Source: CAD feature listing. Evaluate the final solid. Frame: model axes, mm. A direction names the side the tool comes from. Give positions to 0.01 mm unless a question says otherwise; leave off trailing zeros. Loops run counter-clockwise (first coordinate to the right, second up) from the corner with the lowest first, then second, coordinate; pieces in that order, holes last. Notation, with made-up numbers: (76.25, -2.5) - (114.25, -2.5) arc R11 ccw to (114.25, 11.5) - close; hole circle Ø11 at (26, -38). An arc over 180 degrees is marked (long way). Write each question's results on one line, items separated by ' | '. Start each with the question number.
(1) Pull-direction query (Y, two-part tool) for faces 1 (the flat face through (3, -1, 11.75)), 2 (the flat face through (-2.89, 8.54, 0.49)), 3 (the flat face through (8.84, -1.77, 0.49)); classes: pulls with the +Y half, pulls with the -Y half, needs draft (parallel to the pull), parting line crosses it, or undercut.
(2) Cut plane C-C on z = 22.5. Return the cut outline in (x, y), then the cut area to 3 significant figures.
(3) Cut plane B-B on z = 14. Return the cut outline in (x, y), then the cut area to 3 significant figures.
(4) Cut plane A-A on z = 9.75. Return the cut outline in (x, y), then the cut area to 3 significant figures.
(5) Material intervals for line 1 along Y through (x, z) = (0, 20.75); line 2 along Y through (x, z) = (0, 4.25); line 3 along Z through (x, y) = (3, 1.75), sorted ascending. Write a range as [from, to].
(6) Contact query for flat-ended pins moving along their axis: pin 1 (1.5 mm diameter, centred on y = -3.5, z = 6.5, fed in from +X); pin 2 (2 mm diameter, centred on x = -4.5, y = 7.5, fed in from +Z); pin 3 (9 mm diameter, centred on x = -1, y = -1.5, fed in from -Z); pin 4 (3.5 mm diameter, centred on x = 0, y = 0, fed in from +Z). Output: stop coordinate, or through.
(7) Reachability of faces 4 (the cylindrical face through (-1.08, 4.88, 21.44)), 5 (the cylindrical face through (0.75, 5.7, 6.3)), 6 (the flat face through (3.2, -8.97, 7.64)) from +Z, -Z, +X, -X, +Y, -Y: full face, straight path, thin tool, end or side. Return the list, or none.
Autodesk Inventor part; units mm, degrees
ref_plane "Work Plane1" through (0, 0, 16.51) normal (0, 0, 1) x (1, 0, 0)
ref_plane "YZ Plane" through (0, 0, 0) normal (1, 0, 0) x (0, 1, 0)
ref_plane "XZ Plane" through (0, 0, 0) normal (0, 1, 0) x (-1, 0, 0)
sketch "Sketch1" plane through (0, 0, 0) normal (0, 0, 1) x (1, 0, 0)
  line L0 (2.0695, 10.8021) -> (10.3896, 3.6088)
  line L1 (10.3896, 3.6088) -> (8.3201, -7.1932)
  line L2 (8.3201, -7.1932) -> (-2.0695, -10.8021)
  line L3 (-2.0695, -10.8021) -> (-10.3896, -3.6088)
  line L4 (-10.3896, -3.6088) -> (-8.3201, 7.1932)
  line L5 (-8.3201, 7.1932) -> (2.0695, 10.8021)
  point P0 (0, 0)
  point P1 (0, 0)
  dimension "d0" = 19.05
extrude "Extrusion1" add sketch "Sketch1" along normal blind 14.478
ref_plane "Work Plane1" through (0, 0, 16.51) normal (0, 0, 1) x (1, 0, 0)
sketch "Sketch2" plane through (0, 0, 16.51) normal (0, 0, 1) x (1, 0, 0)
  circle A0 centre (0, 0) radius 5
  dimension "d4" = 10
sketch "Sketch3" plane through (0, 0, 14.478) normal (0, 0, 1) x (1, 0, 0)
  line L0 (10.3896, 3.6088) -> (8.3201, -7.1932)
  line L1 (2.0695, 10.8021) -> (10.3896, 3.6088)
  line L2 (-8.3201, 7.1932) -> (2.0695, 10.8021)
  line L3 (-10.3896, -3.6088) -> (-8.3201, 7.1932)
  line L4 (-2.0695, -10.8021) -> (-10.3896, -3.6088)
  line L5 (8.3201, -7.1932) -> (-2.0695, -10.8021)
loft "Loft1" add profiles "Sketch3", "Sketch2"
extrude "Extrusion2" add sketch "Sketch2" along normal blind 10
sketch "Sketch4" plane through (0, 0, 0) normal (0, 0, -1) x (-1, 0, 0)
  circle A0 centre (0, 0) radius 5.75
  dimension "d11" = 11.5
extrude "Extrusion3" cut sketch "Sketch4" against normal blind 11.75
sketch "Sketch5" plane through (0, 0, 11.75) normal (0, 0, -1) x (-1, 0, 0)
  circle A0 centre (0, 0) radius 2.75
  dimension "d14" = 5.5
extrude "Extrusion4" cut sketch "Sketch5" against normal blind 19
thread "Thread1"
thread "Thread2"
chamfer "Chamfer1" distance 1 angle 45 7 edges at (9.3549, -1.7922, 0) (6.2295, 7.2055, 0) (-3.1253, 8.9977, 0) (-9.3549, 1.7922, 0) (-6.2295, -7.2055, 0) (3.1253, -8.9977, 0) (5.75, 0, 0)
properties part number "222P-4-2"
Ans:
1) face 1: undercut | face 2: pulls with the +Y half | face 3: pulls with the -Y half
2) outline: circle Ø10 at (0, 0); hole circle Ø5.5 at (0, 0) | area: 54.8 mm^2
3) outline: (-10.39, -3.61) - (-2.07, -10.8) - (8.32, -7.19) - (10.39, 3.61) - (2.07, 10.8) - (-8.32, 7.19) - close; hole circle Ø5.5 at (0, 0) | area: 291 mm^2
4) outline: (-10.39, -3.61) - (-2.07, -10.8) - (8.32, -7.19) - (10.39, 3.61) - (2.07, 10.8) - (-8.32, 7.19) - close; hole circle Ø11.5 at (0, 0) | area: 210 mm^2
5) line 1: [-5, -2.75], [2.75, 5] | line 2: [-10.08, -5.75], [5.75, 10.08] | line 3: [11.75, 26.51]
6) pin 1: x = 9.17 | pin 2: z = 15.34 | pin 3: z = 0.45 | pin 4: through
7) face 4: +Z | face 5: -Z | face 6: +Z, -Z, +X, -Y
